Here's how the part is built. I have some questions about the finished solid (model axes, mm). A direction names the side the tool comes from. Round coordinates to 2 decimals unless told otherwise and drop trailing zeros. Write each loop counter-clockwise with the first axis right and the second up, starting at its lowest first coordinate (ties: lowest second). Pieces come first, ordered by that corner, then holes. Notation, with made-up numbers: (61.5, 25.25) - (71.5, 25.25) arc R20 ccw to (71.5, 35.25) - close; hole circle Ø4 at (-2.5, 48). An arc over 180 degrees is marked (long way). Write item = value, one per line. Start each with the question number.
Item 1: For P1, Ø4, axis at y = 2, z = 28.5, coming from the +X side; P2, Ø1.2, axis at x = -26, y = 1.5, coming from the +Z side; P3, Ø1.5, axis at x = 23.5, y = 3, coming from the -Z side, each with a flat end and sliding along its axis, tell me the tip position at first contact or that it passes through.
Item 2: If we section it at D-D (x = 12.5): Please give me the cut outline in (y, z), and give its area (3 significant figures).
Item 3: If we section it at A-A (x = 0): Please give me the cut outline in (y, z), and give its area (3 significant figures).
Item 4: Thinking about a two-plate mould opening in Z: for faces 4 (the face through (-19.38, 2.03, 14.48)), 5 (the face through (1.515, 1.972, -49.977)), 6 (the face through (-38.22, 1.97, 24.62)), 7 (the face through (27, -4, 17)), which applies, pulls with the +Z half, pulls with the -Z half, needs draft (parallel to the pull), parting line crosses it, or undercut?
Item 5: If we section it at C-C (y = -1.5): Please give me the cut outline in (x, z).
Item 6: Which directions (+Z, -Z, +X, -X, +Y, -Y) give clear straight access to the entire face, cutting with the end or side of a thin tool? Please do faces 1 (the face through (-7.5, 2, 28)), 2 (the face through (-16.175, 2.028, -18.687)), 3 (the face through (-0.521, -1.972, -31.034)).
Item 7: If I drill on line 1 along Z through (x, y) = (0, -2); line 2 along Y through (x, z) = (-40.5, -26.5); line 3 along X through (y, z) = (3.75, -6), over which ranges is the centre line in solid material (lowest first)? Write a range as [from, to].
Item 8: If we section it at B-B (z = 0): Please give me the cut outline in (x, y), and give its area (3 significant figures).
```python
from build123d import *

# Parameters (mm, degrees)
SKETCH1_R           = 50
BOSS_EXTRUDE1_DEPTH = 4
CUT_EXTRUDE1_START  = -1
SKETCH2_R           = 3
CUT_EXTRUDE1_DEPTH  = 6
CIRPATTERN1_COUNT   = 3
SKETCH3_R           = 4
BOSS_EXTRUDE3_DEPTH = 4
SKETCH4_R           = 3
CUT_EXTRUDE2_DEPTH  = 5
CIRPATTERN2_COUNT   = 3
CUT_EXTRUDE4_DEPTH  = 5
CUT_EXTRUDE5_DEPTH  = 9


with BuildPart() as part:
    # Sketch1 → Boss-Extrude1 (new body)
    with BuildSketch(Plane(origin=(0, 0, 0), x_dir=(1, 0, 0), z_dir=(0, 1, 0))):
        Circle(SKETCH1_R)
    extrude(amount=BOSS_EXTRUDE1_DEPTH)

    # Sketch2 → Cut-Extrude1 (cut)
    with BuildSketch(Plane(origin=(0, 0, 0), x_dir=(1, 0, 0), z_dir=(0, 1, 0)).offset(CUT_EXTRUDE1_START)):
        with Locations((0, 35)):
            Circle(SKETCH2_R)
    cut_extrude1 = extrude(amount=CUT_EXTRUDE1_DEPTH, mode=Mode.SUBTRACT)

    # CirPattern1: Cut-Extrude1 ×3 about axis
    cirpattern1_axis = Axis((0, 0, 0), (0, 1, 0))
    for i in range(1, CIRPATTERN1_COUNT):
        add(cut_extrude1.rotate(cirpattern1_axis, i * 360 / CIRPATTERN1_COUNT), mode=Mode.SUBTRACT)

    # Sketch3 → Boss-Extrude3 (add)
    with BuildSketch(Plane.XZ):
        with Locations((0, -35)):
            Circle(SKETCH3_R)
    boss_extrude3 = extrude(amount=BOSS_EXTRUDE3_DEPTH)

    # Sketch4 → Cut-Extrude2 (cut, through all)
    with BuildSketch(Plane.XZ):
        with Locations((0, -35)):
            Circle(SKETCH4_R)
    cut_extrude2 = extrude(amount=CUT_EXTRUDE2_DEPTH, mode=Mode.SUBTRACT)

    # CirPattern2: Boss-Extrude3, Cut-Extrude2 ×3 about axis
    cirpattern2_axis = Axis((0, 0, 0), (0, 1, 0))
    for i in range(1, CIRPATTERN2_COUNT):
        add(boss_extrude3.rotate(cirpattern2_axis, i * 360 / CIRPATTERN2_COUNT))
        add(cut_extrude2.rotate(cirpattern2_axis, i * 360 / CIRPATTERN2_COUNT), mode=Mode.SUBTRACT)

    # Sketch5 → Cut-Extrude4 (cut, through all)
    with BuildSketch(Plane(origin=(0, 0, 0), x_dir=(1, 0, 0), z_dir=(0, 1, 0))):
        with BuildLine():
            Line((-36, -24.1), (-6, -24.1))
            ThreePointArc((-6, -24.1), (-5, -25.1), (-6, -26.1))
            Line((-6, -26.1), (-7.5, -26.1))
            Line((-7.5, -26.1), (-7.5, -29.8))
            Line((-7.5, -29.8), (7.5, -29.8))
            Line((7.5, -29.8), (7.5, -26.1))
            Line((7.5, -26.1), (6, -26.1))
            ThreePointArc((6, -26.1), (5, -25.1), (6, -24.1))
            Line((6, -24.1), (36, -24.1))
            ThreePointArc((36, -24.1), (38.18825044, -24.604273138), (39.935110512, -26.015375995))
            Line((39.935110512, -26.015375995), (41.455250321, -27.954645783))
            ThreePointArc((41.455250321, -27.954645783), (0, -50), (-41.455250321, -27.954645783))
            Line((-41.455250321, -27.954645783), (-39.935110512, -26.015375995))
            ThreePointArc((-39.935110512, -26.015375995), (-38.18825044, -24.604273138), (-36, -24.1))
        make_face()
    extrude(amount=CUT_EXTRUDE4_DEPTH, mode=Mode.SUBTRACT)

    # Sketch6 → Cut-Extrude5 (cut, through all)
    with BuildSketch(Plane(origin=(0, 4, 0), x_dir=(1, 0, 0), z_dir=(0, 1, 0))):
        with BuildLine():
            Line((-30.3, -7.35), (-30.3, 16.65))
            Line((-30.3, 16.65), (-17.886696873, 16.65))
            ThreePointArc((-17.886696873, 16.65), (-16.149299311, 18.715120553), (-14.217848391, 20.6))
            Line((-14.217848391, 20.6), (22.217848391, 20.6))
            ThreePointArc((22.217848391, 20.6), (31.499084727, 0.224363896), (22.5515498, -20.3))
            Line((22.5515498, -20.3), (-14.5515498, -20.3))
            ThreePointArc((-14.5515498, -20.3), (-19.437717402, -14.384832394), (-22.499575468, -7.35))
            Line((-22.499575468, -7.35), (-30.3, -7.35))
        make_face()
    extrude(amount=-CUT_EXTRUDE5_DEPTH, mode=Mode.SUBTRACT)


solid = part.part
```
Reply:
q1.P1 = 42.4
q1.P2 = 24.1
q1.P3 = -44.52
q2.outline = (0, -48.41) - (4, -48.41) - (4, -20.6) - (0, -20.6) - close; (0, 20.3) - (4, 20.3) - (4, 24.1) - (0, 24.1) - close
q2.area = 126 mm2
q3.outline = (-4, -39) - (0, -39) - (0, -50) - (4, -50) - (4, -38) - (-4, -38) - close; (-4, -32) - (4, -32) - (4, -20.6) - (0, -20.6) - (0, -31) - (-4, -31) - close; (0, 20.3) - (4, 20.3) - (4, 29.8) - (0, 29.8) - close
q3.area = 140 mm2
q4.face_4 = undercut
q4.face_5 = parting line crosses it
q4.face_6 = pulls with the +Z half
q4.face_7 = needs draft
q5.outline = circle Ø8 at (-30.31, 17.5); circle Ø8 at (0, -35); circle Ø8 at (30.31, 17.5); hole circle Ø6 at (-30.31, 17.5); hole circle Ø6 at (0, -35); hole circle Ø6 at (30.31, 17.5)
q6.face_1 = +Z, +Y, -Y
q6.face_2 = +Y, -Y
q6.face_3 = -Y
q7.line_1 = [-39, -38], [-32, -31]
q7.line_2 = [0, 4]
q7.line_3 = [-49.64, -30.3], [30.84, 49.64]
q8.outline = (-50, 0) - (-30.3, 0) - (-30.3, 4) - (-50, 4) - close; (31.5, 0) - (50, 0) - (50, 4) - (31.5, 4) - close
q8.area = 153 mm2
